from build123d import *

# Parameters (mm, degrees)
SKETCH1_W           = 22
SKETCH1_H           = 28.216692514
SKETCH1_R           = 1.315
BOSS_EXTRUDE1_DEPTH = 1.8
SKETCH2_W           = 5.08
SKETCH2_H           = 5.08
BOSS_EXTRUDE2_DEPTH = 0.79375
BOSS_EXTRUDE3_START = -1.8
SKETCH3_W           = 7.62
SKETCH3_H           = 2.54
SKETCH3_W_2         = 20.32
SKETCH3_H_2         = 5.08
BOSS_EXTRUDE3_DEPTH = 5.08


with BuildPart() as part:
    # Sketch1 → Boss-Extrude1 (new body)
    with BuildSketch(Plane(origin=(0, 0, 0), x_dir=(1, 0, 0), z_dir=(0, 1, 0))):
        with Locations((0, 6.545846257)):
            Rectangle(SKETCH1_W, SKETCH1_H)
        with Locations((-9, 5.5625)):
            Circle(SKETCH1_R, mode=Mode.SUBTRACT)
        with Locations((9, 5.5625)):
            Circle(SKETCH1_R, mode=Mode.SUBTRACT)
        with Locations((9, -5.5625)):
            Circle(SKETCH1_R, mode=Mode.SUBTRACT)
        with Locations((-9, -5.5625)):
            Circle(SKETCH1_R, mode=Mode.SUBTRACT)
    extrude(amount=BOSS_EXTRUDE1_DEPTH)

    # Sketch2 → Boss-Extrude2 (add)
    with BuildSketch(Plane(origin=(0, 1.8, 0), x_dir=(1, 0, 0), z_dir=(0, 1, 0))):
        Rectangle(SKETCH2_W, SKETCH2_H)
    extrude(amount=BOSS_EXTRUDE2_DEPTH)

    # Sketch3 → Boss-Extrude3 (add)
    with BuildSketch(Plane(origin=(0, 0, 0), x_dir=(-1, 0, 0), z_dir=(0, -1, 0)).offset(BOSS_EXTRUDE3_START)):
        with Locations((-1.27, 10.924192514)):
            Rectangle(SKETCH3_W, SKETCH3_H)
        with Locations((0, 17.274192514)):
            Rectangle(SKETCH3_W_2, SKETCH3_H_2)
    extrude(amount=-BOSS_EXTRUDE3_DEPTH)


solid = part.part
For this review, take the finished solid that the model builds, in its own axes (mm). A direction names the side the tool comes from. Round coordinates to 2 decimals unless told otherwise and drop trailing zeros. Order: outer loops, then holes, each group sorted by start corner. A loop starts at its lowest first (then second) coordinate and runs counter-clockwise, first axis right, second up. Notation, with made-up numbers: M 86,-9 L 145,-9 A25 cw 145,4 Z; hole C 62,34.25 d10. An arc over 180 degrees is marked long. Use a Markdown table: item, result. Add a question column.
Item 1: Tool access review of faces 5 (the flat face through (0, 4, -14.734)), 6 (the flat face through (5.08, 4, -11)), 7 (the flat face through (0, 4, -19.814)): name each direction out of +Z, -Z, +X, -X, +Y, -Y from which nothing blocks a thin tool from reaching the whole face with its end or side.
Item 2: Add section D-D, the plane z = -11.5. Give the boundary of the cut face in (x, y), then the cut area to 3 significant figures.
Item 3: Add section B-B, the plane x = 9. Give the boundary of the cut face in (y, z).
Item 4: Add section C-C, the plane z = -6. Give the boundary of the cut face in (x, y), then the cut area to 3 significant figures.
Item 5: To check wall thickness, follow line 1 along Z through (x, y) = (-9, 1.05); line 2 along Y through (x, z) = (10.25, -15); line 3 along Z through (x, y) = (6.75, 4.5). State the ranges of each line that lie inside material, in increasing order.
Item 6: Mouldability with a two-part tool opening along Z and no side actions: class faces 1 (the flat face through (0, 1, -20.654)), 2 (the flat face through (1, 4, -12.194)), 3 (the flat face through (0, 1, 7.562)), 4 (the flat face through (0, 6.88, -17)) as released by +Z, released by -Z, zero draft, split by the parting line, or undercut.
Item 7: Insertion check: pin 1 (4 mm diameter, centred on x = 2, y = 4.5, fed in from +Z); pin 2 (4 mm diameter, centred on y = 3.5, z = -17.5, fed in from -X); pin 3 (1.3 mm diameter, centred on y = 5.5, z = -10.5, fed in from +X); pin 4 (1.3 mm diameter, centred on y = 5.5, z = -10.5, fed in from -X). Each pin has a flat end and moves straight along its axis. Give the tip position at first contact, or say it passes through.
Item 8: Add section A-A, the plane y = 3. Give the boundary of the cut face in (x, z).
Geometry results:
| question | item | result |
|---|---|---|
| 1 | face 5 | +X, -X, +Y |
| 1 | face 6 | +Z, +X, +Y |
| 1 | face 7 | -Z, +X, -X, +Y |
| 2 | outline | M -11,0 L 11,0 L 11,1.8 L 5.08,1.8 L 5.08,6.88 L -2.54,6.88 L -2.54,1.8 L -11,1.8 Z |
| 2 | area | 78.3 mm² |
| 3 | outline | M 0,-20.65 L 1.8,-20.65 L 1.8,-19.81 L 6.88,-19.81 L 6.88,-14.73 L 1.8,-14.73 L 1.8,-6.88 L 0,-6.88 Z; M 0,-4.25 L 1.8,-4.25 L 1.8,4.25 L 0,4.25 Z; M 0,6.88 L 1.8,6.88 L 1.8,7.56 L 0,7.56 Z |
| 4 | outline | M -11,0 L -10.24,0 L -10.24,1.8 L -11,1.8 Z; M -7.76,0 L 7.76,0 L 7.76,1.8 L -7.76,1.8 Z; M 10.24,0 L 11,0 L 11,1.8 L 10.24,1.8 Z |
| 4 | area | 30.7 mm² |
| 5 | line 1 | z = -20.65 to -6.88, -4.25 to 4.25, 6.88 to 7.56 |
| 5 | line 2 | y = 0 to 1.8 |
| 5 | line 3 | z = -19.81 to -14.73 |
| 6 | face 1 | released by -Z |
| 6 | face 2 | undercut |
| 6 | face 3 | released by +Z |
| 6 | face 4 | zero draft |
| 7 | pin 1 | stops at z = 2.54 |
| 7 | pin 2 | stops at x = -11 |
| 7 | pin 3 | stops at x = 5.08 |
| 7 | pin 4 | stops at x = -2.54 |
| 8 | outline | M -10.16,-19.81 L 10.16,-19.81 L 10.16,-14.73 L -10.16,-14.73 Z; M -2.54,-12.19 L 5.08,-12.19 L 5.08,-9.65 L -2.54,-9.65 Z |
